Geometry: final body of the model. Coordinates: model frame, mm. Face numbers are marked on the shaded views. Round coordinates to 2 decimals unless told otherwise and drop trailing zeros. Loops run counter-clockwise (first coordinate to the right, second up) from the corner with the lowest first, then second, coordinate; pieces in that order, holes last. Notation, with made-up numbers: (-10.75, 9) - (40.25, 9) arc R10 ccw to (40.25, 14) - close; hole circle Ø3 at (23, 50). An arc over 180 degrees is marked (long way). Answer in a Markdown table with one row per item. Add a question column.
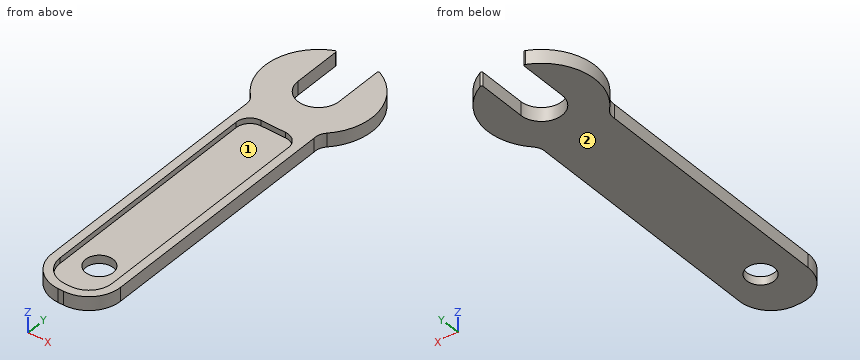
from build123d import *

# Parameters (mm, degrees)
SALIENTE_EXTRUIR1_DEPTH = 10
REDONDEO1_R             = 10
CORTAR_EXTRUIR1_DEPTH   = 4
CROQUIS4_R              = 10
CORTAR_EXTRUIR2_DEPTH   = 10


with BuildPart() as part:
    # Croquis1 → Saliente-Extruir1 (new body)
    with BuildSketch(Plane.XY):
        with BuildLine():
            Line((16.349667964, 100), (25, 100))
            Line((25, 100), (25, -77))
            ThreePointArc((25, -77), (18.263455967, -93.263455967), (2, -100))
            Line((2, -100), (-2, -100))
            ThreePointArc((-2, -100), (-18.263455967, -93.263455967), (-25, -77))
            Line((-25, -77), (-25, 100))
            Line((-25, 100), (-16.349667964, 100))
            ThreePointArc((-16.349667964, 100), (-38.999980166, 135.368129777), (-16.421052632, 170.781873976))
            ThreePointArc((-16.421052632, 170.781873976), (-15.461972413, 170.717764999), (-15, 169.874837769))
            Line((-15, 169.874837769), (-15, 135.40746189))
            ThreePointArc((-15, 135.40746189), (0, 120.40746189), (15, 135.40746189))
            Line((15, 135.40746189), (15, 169.874837769))
            ThreePointArc((15, 169.874837769), (15.461972413, 170.717764999), (16.421052632, 170.781873976))
            ThreePointArc((16.421052632, 170.781873976), (38.999980166, 135.368129777), (16.349667964, 100))
        make_face()
    extrude(amount=SALIENTE_EXTRUIR1_DEPTH)

    # Redondeo1
    # the kernel refuses this fillet: 10 mm, written as the material it adds along each edge
    with BuildSketch(Plane(origin=(-16.349667964, 100, 0), x_dir=(-1, 0, 0), z_dir=(0, 0, 1))) as redondeo1_piece_1:
        with BuildLine():
            CenterArc((18.594262382, -1.057473068), REDONDEO1_R, 173.929776198, 50.579134401)
            Line((11.462848025, -8.067674869), (11.320219738, -8.207878905))
            ThreePointArc((11.320219738, -8.207878905), (5.981746269, -3.678170401), (-0.083844451, -0.181576728))
            Line((-0.083844451, -0.181576728), (0, 0.2))
            ThreePointArc((0, 0.2), (4.325166018, 0.2), (8.451453429, 0.021149461))
            Line((8.451453429, 0.021149461), (8.650332036, 0))
        make_face()
    extrude(amount=10)
    with BuildSketch(Plane(origin=(16.349667964, 100, 0), x_dir=(0.8177652445483508, 0.5755519132178922, 0), z_dir=(0, 0, 1))) as redondeo1_piece_2:
        with BuildLine():
            CenterArc((15.814372171, -9.837198566), REDONDEO1_R, 100.352797219, 50.579134401)
            Line((7.073940893, -4.978715153), (6.899132268, -4.881545485))
            ThreePointArc((6.899132268, -4.881545485), (3.421860064, -2.652910626), (-0.115110383, -0.163553049))
            Line((-0.115110383, -0.163553049), (0.035941755, 0.196743971))
            ThreePointArc((0.035941755, 0.196743971), (7.008642212, -0.434925592), (13.98134267, 0.196743971))
            Line((13.98134267, 0.196743971), (14.017284425, 0))
        make_face()
    extrude(amount=10)

    # Croquis3 → Cortar-Extruir1 (cut)
    with BuildSketch(Plane.XY.offset(10)):
        with BuildLine():
            Line((-2, -94), (2, -94))
            ThreePointArc((2, -94), (14.02081528, -89.02081528), (19, -77))
            Line((19, -77), (19, 84))
            ThreePointArc((19, 84), (16.071067812, 91.071067812), (9, 94))
            Line((9, 94), (-9, 94))
            ThreePointArc((-9, 94), (-16.071067812, 91.071067812), (-19, 84))
            Line((-19, 84), (-19, -77))
            ThreePointArc((-19, -77), (-14.02081528, -89.02081528), (-2, -94))
        make_face()
    extrude(amount=-CORTAR_EXTRUIR1_DEPTH, mode=Mode.SUBTRACT)

    # Croquis4 → Cortar-Extruir2 (cut)
    with BuildSketch(Plane.XY.offset(6)):
        with Locations((0, -64.903172803)):
            Circle(CROQUIS4_R)
    extrude(amount=-CORTAR_EXTRUIR2_DEPTH, mode=Mode.SUBTRACT)


solid = part.part
1) Pull-direction query (Y, two-part tool) for the marked faces 1 and 2; classes: pulls with the +Y half, pulls with the -Y half, needs draft (parallel to the pull), parting line crosses it, or undercut.
2) Section D-D, the plane x = -32.5. Return the cut outline in (y, z), and give its area (3 significant figures).
3) Section C-C, the plane z = 2.75. Return the cut outline in (x, y).
4) Section A-A, the plane y = 123. Return the cut outline in (x, z).
5) Material intervals for line 1 along Y through (x, z) = (0, 3.2); line 2 along X through (y, z) = (-72.5, 7.5); line 3 along X through (y, z) = (76, 3.25), sorted ascending. Write a range as from..to.
6) Contact query for flat-ended pins moving along their axis: pin 1 Ø5 at (y, z) = (47, 6) entering from -X; pin 2 Ø1.2 at (x, z) = (-3, 9) entering from -Y; pin 3 Ø3 at (y, z) = (46.5, 6) entering from +X; pin 4 Ø1 at (x, y) = (-13.5, 142.5) entering from -Z. Output: stop coordinate, or through.
7) Section B-B, the plane y = 80.5. Return the cut outline in (x, z).
Evaluation:
| question | item | result |
|---|---|---|
| 1 | face 1 | undercut |
| 1 | face 2 | needs draft |
| 2 | outline | (113.85, 0) - (156.97, 0) - (156.97, 10) - (113.85, 10) - close |
| 2 | area | 431 mm² |
| 3 | outline | (-27.81, 108.07) arc R10 cw to (-25, 100) - (-25, -77) arc R23 ccw to (-2, -100) - (2, -100) arc R23 ccw to (25, -77) - (25, 100) arc R10 cw to (27.81, 108.07) arc R39 ccw to (16.42, 170.78) arc R1 ccw to (15, 169.87) - (15, 135.41) arc R15 cw to (-15, 135.41) - (-15, 169.87) arc R1 ccw to (-16.42, 170.78) arc R39 ccw to start; hole circle Ø20 at (0, -64.9) |
| 4 | outline | (-36.97, 0) - (-8.43, 0) - (-8.43, 10) - (-36.97, 10) - close; (8.43, 0) - (36.97, 0) - (36.97, 10) - (8.43, 10) - close |
| 5 | line 1 | y = -100..-74.9, -54.9..120.41 |
| 5 | line 2 | x = -25..-19, 19..25 |
| 5 | line 3 | x = -25..25 |
| 6 | pin 1 | stops at x = -25 |
| 6 | pin 2 | stops at y = -100 |
| 6 | pin 3 | stops at x = 25 |
| 6 | pin 4 | passes through |
| 7 | outline | (-25, 0) - (25, 0) - (25, 10) - (19, 10) - (19, 6) - (-19, 6) - (-19, 10) - (-25, 10) - close |
